Could you check a few things on this model? Use its own coordinates, in mm. Round coordinates to 2 decimals unless told otherwise and drop trailing zeros. Write each loop counter-clockwise with the first axis right and the second up, starting at its lowest first coordinate (ties: lowest second). Pieces come first, ordered by that corner, then holes. Notation, with made-up numbers: (-39.75, 16.5) -> (-11.75, 16.5) arc R13 ccw to (-11.75, 37.5) -> close; hole circle Ø8 at (37, -19.5). An arc over 180 degrees is marked (long way). Answer as CSV lines item,"result". Start each with the question number.
Q1. If we mould it in two halves opening along X, with no side actions, what happens to faces 1 (the flat face through (10, 3.048, -10)), 2 (the flat face through (8, 2.54, -8)), 3 (the flat face through (15.24, 1, -8)), 4 (the cylindrical face through (7.07, 2.8, -5.14))? For each: pulls with the +X half, pulls with the -X half, needs draft (parallel to the pull), parting line crosses it, or undercut.
Q2. Imagine slicing it at B-B on x = 11. Please give me the cut outline in (y, z).
Q3. If I drill on line 1 (Z direction, x = 7.62, y = 2.9); line 2 (X direction, y = 2.9, z = -7.62); line 3 (X direction, y = 2.85, z = -11.25), over which ranges is the centre line in solid material (lowest first)? Write a range as [from, to].
Q4. Imagine slicing it at D-D on z = -13. Please give me the cut outline in (x, y), and give its area (3 significant figures).
Q5. Imagine slicing it at A-A on z = -7.62. Please give me the cut outline in (x, y).
Q6. Will this pin go through, and if not, where does the flat tip stop? pin 1 Ø3 at (x, z) = (7.62, -7.62) entering from +Y.
Q7. Imagine slicing it at C-C on x = 7.62. Please give me the cut outline in (y, z), and give its area (3 significant figures).
from build123d import *

# Parameters (mm, degrees)
SKETCH1_W           = 15.24
SKETCH1_H           = 15.24
BOSS_EXTRUDE1_DEPTH = 2.54
SKETCH2_W           = 9.144
SKETCH2_H           = 9.144
BOSS_EXTRUDE2_DEPTH = 3.048
SKETCH3_R           = 2.54
CUT_EXTRUDE1_DEPTH  = 0.508


with BuildPart() as part:
    # Sketch1 → Boss-Extrude1 (new body)
    with BuildSketch(Plane(origin=(0, 0, 0), x_dir=(1, 0, 0), z_dir=(0, 1, 0))):
        with Locations((7.62, 7.62)):
            Rectangle(SKETCH1_W, SKETCH1_H)
    extrude(amount=BOSS_EXTRUDE1_DEPTH)

    # Sketch2 → Boss-Extrude2 (add)
    with BuildSketch(Plane(origin=(0, 0, 0), x_dir=(1, 0, 0), z_dir=(0, 1, 0))):
        with Locations((7.62, 7.62)):
            Rectangle(SKETCH2_W, SKETCH2_H)
    extrude(amount=BOSS_EXTRUDE2_DEPTH)

    # Sketch3 → Cut-Extrude1 (cut)
    with BuildSketch(Plane(origin=(0, 3.048, 0), x_dir=(1, 0, 0), z_dir=(0, 1, 0))):
        with Locations((7.62, 7.62)):
            Circle(SKETCH3_R)
    extrude(amount=-CUT_EXTRUDE1_DEPTH, mode=Mode.SUBTRACT)


solid = part.part
Checks:
1,face 1,"needs draft"
1,face 2,"undercut"
1,face 3,"pulls with the +X half"
1,face 4,"undercut"
2,outline,"(0, -15.24) -> (2.54, -15.24) -> (2.54, -12.19) -> (3.05, -12.19) -> (3.05, -3.05) -> (2.54, -3.05) -> (2.54, 0) -> (0, 0) -> close"
3,line 1,"[-12.19, -10.16], [-5.08, -3.05]"
3,line 2,"[3.05, 5.08], [10.16, 12.19]"
3,line 3,"[3.05, 12.19]"
4,outline,"(0, 0) -> (15.24, 0) -> (15.24, 2.54) -> (0, 2.54) -> close"
4,area,"38.7 mm^2"
5,outline,"(0, 0) -> (15.24, 0) -> (15.24, 2.54) -> (12.19, 2.54) -> (12.19, 3.05) -> (10.16, 3.05) -> (10.16, 2.54) -> (5.08, 2.54) -> (5.08, 3.05) -> (3.05, 3.05) -> (3.05, 2.54) -> (0, 2.54) -> close"
6,pin 1,"y = 2.54"
7,outline,"(0, -15.24) -> (2.54, -15.24) -> (2.54, -12.19) -> (3.05, -12.19) -> (3.05, -10.16) -> (2.54, -10.16) -> (2.54, -5.08) -> (3.05, -5.08) -> (3.05, -3.05) -> (2.54, -3.05) -> (2.54, 0) -> (0, 0) -> close"
7,area,"40.8 mm^2"
